For this review, take the finished solid that the model builds, in its own axes (mm). A direction names the side the tool comes from. Round coordinates to 2 decimals unless told otherwise and drop trailing zeros. Order: outer loops, then holes, each group sorted by start corner. A loop starts at its lowest first (then second) coordinate and runs counter-clockwise, first axis right, second up. Notation, with made-up numbers: M 79,84 L 118,84 A8 ccw 118,97 Z; hole C -3,63.5 d10. An arc over 180 degrees is marked long. Answer as a JSON object with one key per item and string values.
from build123d import *

# Parameters (mm, degrees)
F1_DEPTH = 14
F2_R     = 2.1
F3_DEPTH = 14
F4_R     = 2
F5_R     = 3.1
F6_R     = 2


with BuildPart() as f1:
    # F0 (on Top) → F1 (new body)
    with BuildSketch(Plane.XY):
        Polygon((-65, 18.5), (-75, -19.5), (-57, -19.5), (-50, 4.5), (0, 4.5), (50, 4.5), (57, -19.5), (75, -19.5), (65, 18.5), (0, 18.5), align=None)
    extrude(amount=F1_DEPTH)

    # F2 (on face) → F3 (cut)
    with BuildSketch(Plane.XZ.offset(19.5)):
        with Locations((-62, 7)):
            Circle(F2_R)
        with Locations((62, 7)):
            Circle(F2_R)
    extrude(amount=-F3_DEPTH, mode=Mode.SUBTRACT)

    # F4
    f4_edges = [f1.edges().sort_by_distance(p)[0] for p in [
        (65, 18.5, 7),
        (-65, 18.5, 7),
    ]]
    fillet(f4_edges, radius=F4_R)

    # F5
    f5_edges = [f1.edges().sort_by_distance(p)[0] for p in [
        (50, 4.5, 7),
        (-50, 4.5, 7),
    ]]
    fillet(f5_edges, radius=F5_R)

    # F6
    f6_edges = [f1.edges().sort_by_distance(p)[0] for p in [
        (0, 18.5, 0),
        (-64.679293, 18.083978, 0),
        (-70.196186, -1.245507, 0),
        (64.679293, 18.083978, 0),
        (70.196186, -1.245507, 0),
        (53.8255, -8.616, 0),
        (49.535, 3.88, 0),
        (0, 4.5, 0),
        (-49.535, 3.88, 0),
        (-53.8255, -8.616, 0),
        (-70.196186, -1.245507, 14),
        (-64.679293, 18.083978, 14),
        (0, 18.5, 14),
        (64.679293, 18.083978, 14),
        (70.196186, -1.245507, 14),
        (49.535, 3.88, 14),
        (0, 4.5, 14),
        (53.8255, -8.616, 14),
        (-49.535, 3.88, 14),
        (-53.8255, -8.616, 14),
    ]]
    fillet(f6_edges, radius=F6_R)


solid = f1.part
1) Add section B-B on z = 7. State the section outline as (x, y) points (3 decimals), and give its area (3 significant figures).
Geometry check:
{"outline": "M -75,-19.5 L -64.1,-19.5 L -64.1,-5.5 L -59.9,-5.5 L -59.9,-19.5 L -57,-19.5 L -50.651,2.268 A3.1 cw -47.675,4.5 L 47.675,4.5 A3.1 cw 50.651,2.268 L 57,-19.5 L 59.9,-19.5 L 59.9,-5.5 L 64.1,-5.5 L 64.1,-19.5 L 75,-19.5 L 65.392,17.009 A2 ccw 63.458,18.5 L -63.458,18.5 A2 ccw -65.392,17.009 Z", "area": "2,640 mm²"}
2) Add section D-D on x = -62. State the section outline as (y, z) points, and give its area (3 significant figures).
Geometry check:
{"outline": "M -19.5,0 L 16.5,0 A2 ccw 18.5,2 L 18.5,12 A2 ccw 16.5,14 L -19.5,14 L -19.5,9.1 L -5.5,9.1 L -5.5,4.9 L -19.5,4.9 Z", "area": "471 mm²"}
3) Add section C-C on y = -9. State how many separate pieces and enclosed holes the cut face has, and give its area (3 significant figures).
Geometry check:
{"separate pieces": "2", "enclosed holes": "2", "area": "478 mm²"}
4) Insertion check: P1, Ø1.3, axis at x = -61, z = 6.5, coming from the -Y side; P2, Ø3, axis at x = 3, z = 7, coming from the -Y side; P3, Ø6, axis at y = -14.5, z = 11.5, coming from the +X side; P4, Ø4.5, axis at x = 62.5, z = 8, coming from the -Y side. Each pin has a flat end and moves straight along its axis. Give the tip position at first contact, or say it passes through.
Geometry check:
{"P1": "stops at y = -5.5", "P2": "stops at y = 4.5", "P3": "stops at x = 74.47", "P4": "stops at y = -19.5"}
5) Machinability: for faces 5 (the cylindrical face through (54.53, -8.88, 0.57)), 6 (the cylindrical face through (-54.41, -8.58, 13.4)), 7 (the cylindrical face through (-49.56, 3.86, 7.07)), 8 (the flat face through (62, -5.5, 7)), which of the approach directions +Z, -Z, +X, -X, +Y, -Y give a long, thin tool a straight path to every point of the face, cutting with its end or side? Answer none if there is none.
Geometry check:
{"face 5": "-Z, -Y", "face 6": "+Z, -Y", "face 7": "+Z, -Z, -Y", "face 8": "-Y"}
6) Add section A-A on x = 13. State the section outline as (y, z) points, and give its area (3 significant figures).
Geometry check:
{"outline": "M 4.5,2 A2 ccw 6.5,0 L 16.5,0 A2 ccw 18.5,2 L 18.5,12 A2 ccw 16.5,14 L 6.5,14 A2 ccw 4.5,12 Z", "area": "193 mm²"}
7) Mouldability with a two-part tool opening along X and no side actions: class faces 1 (the cylindrical face through (-54.44, -8.57, 0.57)), 2 (the flat face through (1, 18.5, 7)), 3 (the flat face through (-1, 4.5, 7)), 4 (the cylindrical face through (-69.68, -1.65, 0.57)) as +X half, -X half, draft (parallel to the pull), parting line (faces both ways), or undercut.
Geometry check:
{"face 1": "undercut", "face 2": "draft", "face 3": "undercut", "face 4": "-X half"}
8) For L1, parallel to X at y = -16.5, z = 7.5 (3 decimals); L2, parallel to Z at x = 62, y = -13.5; L3, parallel to Y at x = 43, z = 6.5, list the stretches that pass through material, from the lowest coordinate up.
Geometry check:
{"L1": "x = -74.211 to -64.04, -59.96 to -56.125, 56.125 to 59.96, 64.04 to 74.211", "L2": "z = 0 to 4.9, 9.1 to 14", "L3": "y = 4.5 to 18.5"}
